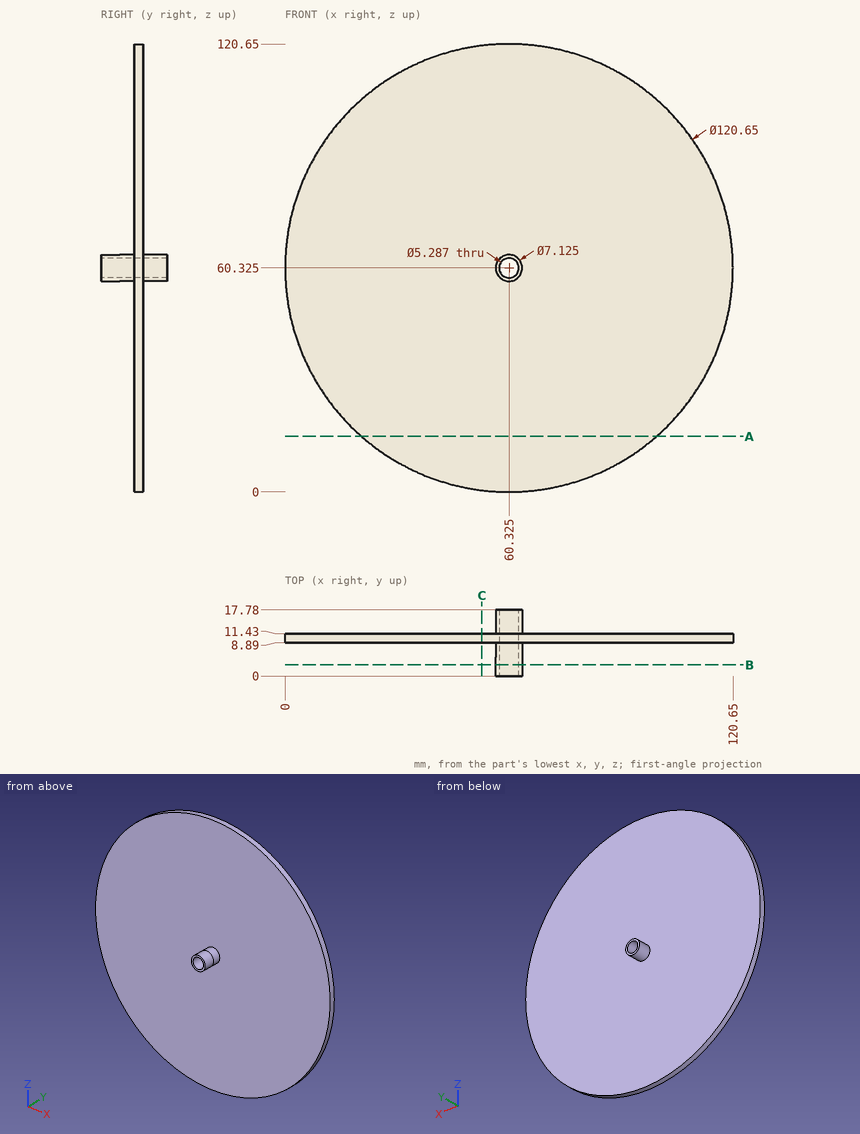
Here's the drawing with two shaded views (mm, measured from the low corner). I have some questions. Coordinates: 2 decimals unless noted, no trailing zeros. Write each loop counter-clockwise with the first axis right and the second up, starting at its lowest first coordinate (ties: lowest second). Pieces come first, ordered by that corner, then holes.
Item 1: I want a section at A-A on z = 15. Write out the boundary of the cut face in (x, y).
Item 2: I want a section at B-B on y = 3. Write out the boundary of the cut face in (x, z) (1 decimal).
Item 3: Will these pins go through, and if not, where does the flat tip stop? pin 1 (8 mm diameter, centred on x = 60.5, y = 5.5, fed in from +Z); pin 2 (2 mm diameter, centred on x = 24, y = 8, fed in from +Z); pin 3 (2 mm diameter, centred on x = 20, z = 38.5, fed in from -Y).
Item 4: If I drill on line 1 (Y direction, x = 90.5, z = 57); line 2 (X direction, y = 11.25, z = 20.5) (1 decimal); line 3 (X direction, y = 10.75, z = 41), over which ranges is the centre line in solid material (lowest first)?
Item 5: I want a section at C-C on x = 53. Write out the boundary of the cut face in (y, z).
Findings below:
1. outline: (20.52, 8.89) - (100.13, 8.89) - (100.13, 11.43) - (20.52, 11.43) - close
2. outline: circle Ø7.1 at (60.3, 60.3); hole circle Ø5.3 at (60.3, 60.3)
3. pin 1: stops at z = 120.65
3. pin 2: stops at z = 108.83
3. pin 3: stops at y = 8.89
4. line 1: y = 8.89 to 11.43
4. line 2: x = 15 to 105.6
4. line 3: x = 3.18 to 117.47
5. outline: (8.89, 0.45) - (11.43, 0.45) - (11.43, 120.2) - (8.89, 120.2) - close
